from build123d import *

# Parameters (mm, degrees)
F1_DEPTH  = 5
F3_DEPTH  = 8
F5_DEPTH  = 5
F6_R      = 12
F7_DEPTH  = 5
F8_R      = 12
F9_DEPTH  = 5
F11_DEPTH = 13.001
F12_R     = 1.5
F13_DEPTH = 18.001
F14_R     = 2.5
F15_DEPTH = 1.5
F16_R     = 2.5
F17_DEPTH = 1.5
F18_R     = 113.2772211927
F19_DEPTH = 12.5


with BuildPart() as f1:
    # F0 (on Right) → F1 (new body)
    with BuildSketch(Plane.YZ):
        with BuildLine():
            ThreePointArc((46.6693164652, 11.5285101896), (24.2181276728, 7.6768989517), (1.4706951967, 8.8790233494))
            ThreePointArc((1.4706951967, 8.8790233494), (-9, 0), (1.4706951967, -8.8790233494))
            ThreePointArc((1.4706951967, -8.8790233494), (24.2181276728, -7.6768989517), (46.6693164652, -11.5285101896))
            ThreePointArc((46.6693164652, -11.5285101896), (62, 0), (46.6693164652, 11.5285101896))
        make_face()
    extrude(amount=F1_DEPTH)

    # F2 (on face) → F3 (join)
    with BuildSketch(Plane.YZ.offset(5)):
        with BuildLine():
            ThreePointArc((46.6693164652, 11.5285101896), (24.2181276728, 7.6768989517), (1.4706951967, 8.8790233494))
            ThreePointArc((1.4706951967, 8.8790233494), (0.7378312326, 8.9697048487), (0, 9))
            Line((0, 9), (0, 7))
            ThreePointArc((0, 7), (3.4468203516, 6.0925716626), (6, 3.6055512755))
            Line((6, 3.6055512755), (12.7617545607, -7.6466884694))
            ThreePointArc((12.7617545607, -7.6466884694), (29.8782372644, -8.1664058525), (46.6693164652, -11.5285101896))
            ThreePointArc((46.6693164652, -11.5285101896), (62, 0), (46.6693164652, 11.5285101896))
        make_face()
    extrude(amount=F3_DEPTH)

    # F4 (on face) → F5 (join)
    with BuildSketch(Plane.YZ.offset(13)):
        with BuildLine():
            ThreePointArc((1.4706951967, 8.8790233494), (0.7378312326, 8.9697048487), (0, 9))
            ThreePointArc((0, 9), (-8.9697048487, -0.7378312326), (1.4706951967, -8.8790233494))
            ThreePointArc((1.4706951967, -8.8790233494), (7.0991420432, -8.1063373261), (12.7617545607, -7.6466884694))
            ThreePointArc((12.7617545607, -7.6466884694), (29.8782372644, -8.1664058525), (46.6693164652, -11.5285101896))
            ThreePointArc((46.6693164652, -11.5285101896), (62, 0), (46.6693164652, 11.5285101896))
            ThreePointArc((46.6693164652, 11.5285101896), (24.2181276728, 7.6768989517), (1.4706951967, 8.8790233494))
        make_face()
    extrude(amount=F5_DEPTH)

    # F6 (on face) → F7 (cut)
    with BuildSketch(Plane.YZ.offset(18)):
        with Locations((50, 0)):
            Circle(F6_R)
    extrude(amount=-F7_DEPTH, mode=Mode.SUBTRACT)

    # F8 (on face) → F9 (cut)
    with BuildSketch(Plane(origin=(0, 0, 0), x_dir=(0, -1, 0), z_dir=(-1, 0, 0))):
        with Locations((-50, 0)):
            Circle(F8_R)
    extrude(amount=-F9_DEPTH, mode=Mode.SUBTRACT)

    # F10 (on face) → F11 (cut, through all)
    with BuildSketch(Plane.YZ.offset(13)):
        with BuildLine():
            Line((54.5, -7.7942286341), (47.6261364576, -11.7628556007))
            ThreePointArc((47.6261364576, -11.7628556007), (61.9405667204, -1.1928396355), (50, 12))
            Line((50, 12), (50, 9))
            ThreePointArc((50, 9), (58.6933324366, 2.3293714059), (54.5, -7.7942286341))
        make_face()
    extrude(amount=-F11_DEPTH, mode=Mode.SUBTRACT)

    # F12 (on face) → F13 (cut, through all)
    with BuildSketch(Plane.YZ.offset(18)):
        Circle(F12_R)
        with Locations((50, 0)):
            Circle(F12_R)
    extrude(amount=-F13_DEPTH, mode=Mode.SUBTRACT)

    # F14 (on face) → F15 (cut)
    with BuildSketch(Plane.YZ.offset(18)):
        Circle(F14_R)
    extrude(amount=-F15_DEPTH, mode=Mode.SUBTRACT)

    # F16 (on face) → F17 (cut)
    with BuildSketch(Plane(origin=(0, 0, 0), x_dir=(0, -1, 0), z_dir=(-1, 0, 0))):
        Circle(F16_R)
    extrude(amount=-F17_DEPTH, mode=Mode.SUBTRACT)

    # F18 (on Top) → F19 (cut, symmetric)
    with BuildSketch(Plane.XY):
        with Locations((-111, 24.070005831)):
            Circle(F18_R)
        with Locations((129, 24.070005831)):
            Circle(F18_R)
    extrude(amount=F19_DEPTH, both=True, mode=Mode.SUBTRACT)


solid = f1.part
Source: CAD feature listing. Evaluate the final solid. Frame: model axes, mm. A direction names the side the tool comes from. Coordinates: 2 decimals unless noted, no trailing zeros. Order: outer loops, then holes, each group sorted by start corner. A loop starts at its lowest first (then second) coordinate and runs counter-clockwise, first axis right, second up.
Item 1: Material intervals for line 1 (Z direction, x = 2.95, y = 0); line 2 (X direction, y = 1.5, z = -6); line 3 (Z direction, x = 1.15, y = 0), sorted ascending.
Output values:
line 1: z = -9 to -1.5, 1.5 to 9
line 2: x = 0.01 to 5, 13 to 17.99
line 3: z = -9 to -2.5, 2.5 to 9
Item 2: Cut plane B-B (y = 42.5). Return loops of the section in (x, z).
Output values:
outline: (0.77, -10.42) - (17.23, -10.42) - (17.23, -9.37) - (13, -9.37) - (13, 9.37) - (17.23, 9.37) - (17.23, 10.42) - (0.77, 10.42) - (0.77, 9.37) - (5, 9.37) - (5, -9.37) - (0.77, -9.37) - close
Item 3: First-contact query: P1, Ø5.5, axis at y = -1, z = 1, coming from the +X side; P2, Ø3, axis at x = 9.5, y = 23.5, coming from the +Z side; P3, Ø10, axis at x = 2.5, z = -9.5, coming from the -Y side; P4, Ø6, axis at y = 47, z = -1, coming from the -X side. Flat tips, straight axial feed; report the tip coordinate or a pass-through.
Output values:
P1: stops at x = 18
P2: stops at z = 7.73
P3: stops at y = -7.79
P4: stops at x = 5
Item 4: Set-up query: faces 1 (the face through (8.944, 9.334, -1.942)), 2 (the face through (9, 0, 8)), 3 (the face through (1.5, 0, -2)). Return all of +Z, -Z, +X, -X, +Y, -Y with unobstructed straight access to the full face (end or side cutting, diameter ignored); none if empty.
Output values:
face 1: -Z, -Y
face 2: +Z, -Z, -Y
face 3: -X
Item 5: Cut plane C-C (x = 14.75). Return loops of the section in (y, z), plus the area to 3 significant figures.
Output values:
outline: (1.47, -8.88) arc R102.5 cw to (46.67, -11.53) arc R12 cw to (46.67, 11.53) arc R102.5 cw to (1.47, 8.88) arc R9 ccw (long way) to start; hole circle Ø3 at (0, 0)
area: 768 mm2
Item 6: Cut plane A-A (z = 0). Count the separate pieces of the cut face and the enclosed holes in it, plus the area to 3 significant figures.
Output values:
separate pieces: 4
enclosed holes: 0
area: 693 mm2
Item 7: Cut plane D-D (z = -4.5). Return loops of the section in (x, y).
Output values:
outline: (0, -7.79) - (5, -7.79) - (5, 10.87) - (13, 10.87) - (13, -7.79) - (18, -7.79) - (18, 1.47) arc R113.28 cw to (16.69, 38.88) - (13, 38.88) - (13, 57.79) - (5, 57.79) - (5, 38.88) - (1.31, 38.88) arc R113.28 cw to (0, 1.47) - close
Item 8: Pull-direction query (Z, two-part tool) for faces 4 (the face through (8.94, 3.4, 6.12)), 5 (the face through (14.77, -1.5, 0.07)), 6 (the face through (13, -1, -2)), 7 (the face through (15, 38, 0)); classes: pulls with the +Z half, pulls with the -Z half, needs draft (parallel to the pull), parting line crosses it, or undercut.
Output values:
face 4: pulls with the -Z half
face 5: undercut
face 6: needs draft
face 7: undercut
